```python
from build123d import *

# Parameters (mm, degrees)
SKETCH1_R           = 11
BOSS_EXTRUDE1_DEPTH = 10
SKETCH2_R           = 20
BOSS_EXTRUDE2_DEPTH = 105
CUT_EXTRUDE1_DEPTH  = 109.742815855
SKETCH5_R           = 7.125
CUT_EXTRUDE2_DEPTH  = 109.742815988
CUT_EXTRUDE3_START  = -105
CUT_EXTRUDE3_DEPTH  = 105


with BuildPart() as part:
    # Sketch1 → Boss-Extrude1 (new body)
    with BuildSketch(Plane.XY):
        Circle(SKETCH1_R)
    extrude(amount=BOSS_EXTRUDE1_DEPTH)

    # Sketch2 → Boss-Extrude2 (add)
    with BuildSketch(Plane(origin=(0, 0, 0), x_dir=(-1, 0, 0), z_dir=(0, 0, -1))):
        Circle(SKETCH2_R)
    extrude(amount=BOSS_EXTRUDE2_DEPTH)

    # Sketch3 → Cut-Extrude1 (cut, through all)
    with BuildSketch(Plane(origin=(0, 0, 0), x_dir=(0, 0, -1), z_dir=(1, 0, 0))):
        with BuildLine():
            Line((139.625, 14.75), (89.625, 14.75))
            ThreePointArc((89.625, 14.75), (75, 0.125), (89.625, -14.5))
            Line((89.625, -14.5), (139.625, -14.5))
            Line((139.625, -14.5), (139.625, 14.75))
        make_face()
    extrude(amount=-CUT_EXTRUDE1_DEPTH, mode=Mode.SUBTRACT)

    # Sketch5 → Cut-Extrude2 (cut, through all)
    with BuildSketch(Plane.ZY):
        with Locations((-90, 0.125)):
            Circle(SKETCH5_R)
    extrude(amount=-CUT_EXTRUDE2_DEPTH, mode=Mode.SUBTRACT)

    # Sketch6 → Cut-Extrude3 (cut)
    with BuildSketch(Plane(origin=(0, 0, -105), x_dir=(-1, 0, 0), z_dir=(0, 0, -1)).offset(CUT_EXTRUDE3_START)):
        with BuildLine():
            Line((-11.346386998, 16.469957562), (-11.346386998, -16.469957562))
            ThreePointArc((-11.346386998, -16.469957562), (-20, 0), (-11.346386998, 16.469957562))
        make_face()
    extrude(amount=CUT_EXTRUDE3_DEPTH, mode=Mode.SUBTRACT)


solid = part.part
```
Can you work these out from the model? Positions are in its coordinate system, mm. A direction names the side the tool comes from. Coordinates: 2 decimals unless noted, no trailing zeros. Loops run counter-clockwise (first coordinate to the right, second up) from the corner with the lowest first, then second, coordinate; pieces in that order, holes last. Notation, with made-up numbers: (-8.75, 10.25) - (32.25, 10.25) arc R8 ccw to (32.25, 14.25) - close; hole circle Ø9 at (72.5, 68.25). An arc over 180 degrees is marked (long way). Use a Markdown table: item, result.
Item 1: I want a section at B-B on x = -2.5. Please give me the cut outline in (y, z) (3 decimals), and give its area (3 significant figures).
Numbers:
| item | result |
|---|---|
| outline | (-19.843, -105) - (-14.5, -105) - (-14.5, -89.625) arc R14.625 cw to (14.75, -89.625) - (14.75, -105) - (19.843, -105) - (19.843, 0) - (10.712, 0) - (10.712, 10) - (-10.712, 10) - (-10.712, 0) - (-19.843, 0) - close |
| area | 3,600 mm2 |
Item 2: We'd pull the mould along Y, two halves only. Please class faces 4 (the face through (0, 0, 10)), 5 (the face through (0, 3.6, -96.5)), 6 (the face through (-19.99, -0.61, -51.76)): released by +Y, released by -Y, zero draft, split by the parting line, or undercut.
Numbers:
| item | result |
|---|---|
| face 4 | zero draft |
| face 5 | undercut |
| face 6 | split by the parting line |
Item 3: I want a section at A-A on y = -5.5. Please give me the cut outline in (x, z) (3 decimals).
Numbers:
| item | result |
|---|---|
| outline | (-19.229, -76.125) - (0, -76.125) - (0, -85.627) - (11.346, -85.627) - (11.346, 0) - (9.526, 0) - (9.526, 10) - (-9.526, 10) - (-9.526, 0) - (-19.229, 0) - close; (0, -105) - (11.346, -105) - (11.346, -94.373) - (0, -94.373) - close |
Item 4: If I drill on probe 1 along Z at (x, y) = (4, -13); probe 2 along Y at (x, z) = (4, -90); probe 3 along X at (y, z) = (14.5, -84), over which ranges is the centre line in solid material (lowest first)? Write a range as from..to.
Numbers:
| item | result |
|---|---|
| probe 1 | z = -105..0 |
| probe 2 | y = -19.6..-7, 7.25..19.6 |
| probe 3 | x = -13.77..11.35 |
Item 5: Will these pins go through, and if not, where does the flat tip stop? pin 1 (9 mm diameter, centred on y = 0, z = -96, fed in from -X); pin 2 (5 mm diameter, centred on y = 7, z = -53.5, fed in from -X); pin 3 (4 mm diameter, centred on x = -9.5, y = 10, fed in from +Z).
Numbers:
| item | result |
|---|---|
| pin 1 | stops at x = 0 |
| pin 2 | stops at x = -19.49 |
| pin 3 | stops at z = 0 |
Item 6: I want a section at D-D on y = 2. Please give me the cut outline in (x, z), and give its area (3 significant figures).
Numbers:
| item | result |
|---|---|
| outline | (-19.9, -75.12) - (0, -75.12) - (0, -83.13) - (11.35, -83.13) - (11.35, 0) - (10.82, 0) - (10.82, 10) - (-10.82, 10) - (-10.82, 0) - (-19.9, 0) - close; (0, -105) - (11.35, -105) - (11.35, -96.87) - (0, -96.87) - close |
| area | 2,750 mm2 |
Item 7: I want a section at C-C on x = 3.5. Please give me the cut outline in (y, z) (3 decimals), and give its area (3 significant figures).
Numbers:
| item | result |
|---|---|
| outline | (-19.691, -105) - (19.691, -105) - (19.691, 0) - (10.428, 0) - (10.428, 10) - (-10.428, 10) - (-10.428, 0) - (-19.691, 0) - close; hole circle Ø14.25 at (0.125, -90) |
| area | 4,180 mm2 |
Item 8: For faces 1 (the face through (-7, 14.75, -97)), 2 (the face through (11.346, 0, -52)), 3 (the face through (-2.38, -10.74, 4.93)), which set-ups out of +Z, -Z, +X, -X, +Y, -Y let a thin tool reach every point of the face, with its end or its side?
Numbers:
| item | result |
|---|---|
| face 1 | -Z, -X |
| face 2 | +Z, -Z, +X, +Y, -Y |
| face 3 | +Z |
